Could you check a few things on this model? Use its own coordinates, in mm. A direction names the side the tool comes from. Give positions to 0.01 mm unless a question says otherwise; leave off trailing zeros. Answer as a JSON object with one key per item and string values. Group by question number.
```python
from build123d import *

# Parameters (mm, degrees)
F0_W     = 69.85
F0_H     = 114.3
F1_DEPTH = 4.826
F2_SIZE  = 4.82599


# Not quite as in the source:
# - a fillet or chamfer is up to 0.001 mm smaller than in the source, because OpenCascade refuses the exact size


with BuildPart() as f1:
    # F0 (on Front) → F1 (new body)
    with BuildSketch(Plane.XZ):
        Rectangle(F0_W, F0_H)
        with BuildLine():
            add(Edge.make_bspline(
                [(-10.16, -5.08), (-13.589, -9.8636666667), (-20.447, -19.431), (-13.589, -28.9983333333), (-10.16, -33.782)],
                knots=[0, 0, 0, 0, 0.5, 1, 1, 1, 1], degree=3))
            Line((-10.16, -5.08), (10.16, -5.08))
            add(Edge.make_bspline(
                [(10.16, -5.08), (13.589, -9.8636666667), (20.447, -19.431), (13.589, -28.9983333333), (10.16, -33.782)],
                knots=[0, 0, 0, 0, 0.5, 1, 1, 1, 1], degree=3))
            Line((10.16, -33.782), (-10.16, -33.782))
        make_face(mode=Mode.SUBTRACT)
        with BuildLine():
            add(Edge.make_bspline(
                [(-10.16, 33.782), (-13.589, 28.9983333333), (-20.447, 19.431), (-13.589, 9.8636666667), (-10.16, 5.08)],
                knots=[0, 0, 0, 0, 0.5, 1, 1, 1, 1], degree=3))
            Line((-10.16, 33.782), (10.16, 33.782))
            add(Edge.make_bspline(
                [(10.16, 33.782), (13.589, 28.9983333333), (20.447, 19.431), (13.589, 9.8636666667), (10.16, 5.08)],
                knots=[0, 0, 0, 0, 0.5, 1, 1, 1, 1], degree=3))
            Line((10.16, 5.08), (-10.16, 5.08))
        make_face(mode=Mode.SUBTRACT)
    extrude(amount=F1_DEPTH)

    # F2 (size 4.826 in the source; OpenCascade refuses exactly that, so slightly less here)
    f2_edges = [f1.edges().sort_by_distance(p)[0] for p in [
        (-34.925, -4.826, 0),
        (0, -4.826, 57.15),
        (34.925, -4.826, 0),
        (0, -4.826, -57.15),
    ]]
    chamfer(f2_edges, length=F2_SIZE)


solid = f1.part
```
(1) Will these pins go through, and if not, where does the flat tip stop? P1, Ø1.5, axis at x = 19.5, y = -2, coming from the +Z side; P2, Ø2, axis at x = -8, y = -1.5, coming from the +Z side; P3, Ø1.4, axis at x = 1.5, y = -2, coming from the +Z side.
(2) If we mould it in two halves opening along Z, with no side actions, what happens to faces 1 (the flat face through (-0.49, -2.45, 54.7)), 2 (the flat face through (0, -2, -5.08)), 3 (the flat face through (0, -4.826, 1))? For each: +Z half, -Z half, draft (parallel to the pull), parting line (faces both ways), or undercut.
(3) I want a section at A-A, the plane x = -7.5. State how many separate pieces and enclosed holes the cut face has, and give its area (3 significant figures).
(4) I need wall thicknesses on L1, parallel to Z at x = -7, y = -3.5; L2, parallel to Z at x = 3, y = -1.3; L3, parallel to X at y = -3.4, z = 21 (3 decimals). Which ranges of each line are inside material? Lowest first, please.
(5) For faces 4 (the flat face through (0, 0, 1)), 5 (the flat face through (0, -2, 5.08)), which set-ups out of +Z, -Z, +X, -X, +Y, -Y let a thin tool reach every point of the face, with its end or its side?
Entries:
{
 "1": {"P1": "z = 55.9", "P2": "z = 56.65", "P3": "z = 55.85"},
 "2": {"face 1": "+Z half", "face 2": "undercut", "face 3": "draft"},
 "3": {"separate pieces": "3", "enclosed holes": "0", "area": "251 mm^2"},
 "4": {"L1": "-53.65 to -33.78, -5.08 to 5.08, 33.78 to 53.65", "L2": "-55.85 to -33.78, -5.08 to 5.08, 33.78 to 55.85", "L3": "-31.525 to -16.9, 16.9 to 31.525"},
 "5": {"face 4": "+Z, -Z, +X, -X, +Y", "face 5": "+Y, -Y"}
}
